```python
from build123d import *

# Parameters (mm, degrees)
SKETCH_1_W          = 25
SKETCH_1_H          = 16
EXTRUDE_1_DEPTH     = 2
SKETCH_2_R          = 0.5
CUT_EXTRUDE_1_DEPTH = 3
SKETCH_3_W          = 1.998432602
SKETCH_3_H          = 1
EXTRUDE_2_DEPTH     = 0.5
SKETCH_4_W          = 4
SKETCH_4_H          = 2
EXTRUDE_3_DEPTH     = 2
SKETCH_5_W          = 1.76862678
SKETCH_5_H          = 1.058923041
EXTRUDE_4_DEPTH     = 1


with BuildPart() as part:
    # 草图1 → 凸台-拉伸1 (new body)
    with BuildSketch(Plane.XY):
        with Locations((12.5, 8)):
            Rectangle(SKETCH_1_W, SKETCH_1_H)
    extrude(amount=EXTRUDE_1_DEPTH)

    # 草图2 → 切除-拉伸1 (cut, through all)
    with BuildSketch(Plane(origin=(0, 0, 0), x_dir=(-1, 0, 0), z_dir=(0, 0, -1))):
        with Locations((-1, 14.4)):
            Circle(SKETCH_2_R)
        with Locations((-1, 11.86)):
            Circle(SKETCH_2_R)
        with Locations((-1, 9.32)):
            Circle(SKETCH_2_R)
        with Locations((-1, 6.78)):
            Circle(SKETCH_2_R)
        with Locations((-1, 4.24)):
            Circle(SKETCH_2_R)
        with Locations((-1, 1.7)):
            Circle(SKETCH_2_R)
    extrude(amount=-CUT_EXTRUDE_1_DEPTH, mode=Mode.SUBTRACT)

    # 草图3 → 凸台-拉伸2 (add)
    with BuildSketch(Plane(origin=(0, 0, 0), x_dir=(-1, 0, 0), z_dir=(0, 0, -1))):
        with Locations((-22.800563102, 10)):
            Rectangle(SKETCH_3_W, SKETCH_3_H)
        with Locations((-22.800563102, 8)):
            Rectangle(SKETCH_3_W, SKETCH_3_H)
        with Locations((-22.800563102, 6)):
            Rectangle(SKETCH_3_W, SKETCH_3_H)
        with Locations((-22.800563102, 4)):
            Rectangle(SKETCH_3_W, SKETCH_3_H)
    extrude(amount=EXTRUDE_2_DEPTH)

    # 草图4 → 凸台-拉伸3 (add)
    with BuildSketch(Plane(origin=(0, 0, 0), x_dir=(-1, 0, 0), z_dir=(0, 0, -1))):
        with Locations((-20, 1)):
            Rectangle(SKETCH_4_W, SKETCH_4_H)
    extrude(amount=EXTRUDE_3_DEPTH)

    # 草图5 → 凸台-拉伸4 (add)
    with BuildSketch(Plane.XZ):
        with Locations((19.9984492, -0.838988802)):
            Rectangle(SKETCH_5_W, SKETCH_5_H)
    extrude(amount=EXTRUDE_4_DEPTH)


solid = part.part
```
Design review of the part built by this model. Coordinates are the model's own, in mm. A direction names the side the tool comes from. Coordinates: 2 decimals unless noted, no trailing zeros. Order: outer loops, then holes, each group sorted by start corner. A loop starts at its lowest first (then second) coordinate and runs counter-clockwise, first axis right, second up. Notation, with made-up numbers: (-19.5, 42) - (-1.5, 42) arc R14 cw to (-1.5, 61) - close; hole circle Ø5 at (15.25, 63). An arc over 180 degrees is marked (long way). Answer in a Markdown table with one row per item.
(1) Consider section B-B on z = 0.65. State the section outline as (x, y) points, plus the area to 3 significant figures.
Checked values:
| item | result |
|---|---|
| outline | (0, 0) - (25, 0) - (25, 16) - (0, 16) - close; hole circle Ø1 at (1, 1.7); hole circle Ø1 at (1, 4.24); hole circle Ø1 at (1, 6.78); hole circle Ø1 at (1, 9.32); hole circle Ø1 at (1, 11.86); hole circle Ø1 at (1, 14.4) |
| area | 395 mm^2 |
(2) For faces 1 (the flat face through (20, -0.5, -0.31)), 2 (the flat face through (20.883, -0.5, -0.8)), 3 (the flat face through (18, 1, -1)), list the 3-axis set-ups (+Z, -Z, +X, -X, +Y, -Y) from which the entire face can be reached by the end or side of a thin tool; tool diameter is ignored.
Checked values:
| item | result |
|---|---|
| face 1 | +Z, +X, -X, -Y |
| face 2 | +Z, -Z, +X, -Y |
| face 3 | -Z, -X, +Y, -Y |
(3) Wall thickness on line 1 along Y through (x, z) = (9.5, 0.6); line 2 along Z through (x, y) = (22, 4.75); line 3 along X through (y, z) = (9, 0.2): over which ranges is each line inside the solid? List them lowest first. Write a range as from..to.
Checked values:
| item | result |
|---|---|
| line 1 | 0..16 |
| line 2 | 0..2 |
| line 3 | 0..0.62, 1.38..25 |
(4) Consider section A-A on y = 1.7. State the section outline as (x, z) points, plus the area to 3 significant figures.
Checked values:
| item | result |
|---|---|
| outline | (0, 0) - (0.5, 0) - (0.5, 2) - (0, 2) - close; (1.5, 0) - (18, 0) - (18, -2) - (22, -2) - (22, 0) - (25, 0) - (25, 2) - (1.5, 2) - close |
| area | 56.0 mm^2 |
(5) Clearance check with flat-ended pins moving along their axes: pin 1 (0.5 mm diameter, centred on x = 22.5, y = 6, fed in from -Z); pin 2 (2 mm diameter, centred on x = 5, z = -0.5, fed in from -Y); pin 3 (0.8 mm diameter, centred on x = 20, y = -0.5, fed in from -Z). State where each tip first meets the part, or that it passes through.
Checked values:
| item | result |
|---|---|
| pin 1 | z = -0.5 |
| pin 2 | y = 0 |
| pin 3 | z = -1.37 |
(6) The part is to be moulded in two halves that separate along Y. For faces 4 (the cylindrical face through (1.108, 11.372, 0.986)), 5 (the flat face through (12, 16, 1)), 6 (the cylindrical face through (1.065, 7.276, 0.986)), 7 (the flat face through (0, 8, 1)), say which applies: released by +Y, released by -Y, zero draft, split by the parting line, or undercut.
Checked values:
| item | result |
|---|---|
| face 4 | undercut |
| face 5 | released by +Y |
| face 6 | undercut |
| face 7 | zero draft |
(7) Consider section D-D on y = 11.86. State the section outline as (x, z) points, plus the area to 3 significant figures.
Checked values:
| item | result |
|---|---|
| outline | (0, 0) - (0.5, 0) - (0.5, 2) - (0, 2) - close; (1.5, 0) - (25, 0) - (25, 2) - (1.5, 2) - close |
| area | 48.0 mm^2 |
(8) Consider section C-C on x = 1. State the section outline as (y, z) points, plus the area to 3 significant figures.
Checked values:
| item | result |
|---|---|
| outline | (0, 0) - (1.2, 0) - (1.2, 2) - (0, 2) - close; (2.2, 0) - (3.74, 0) - (3.74, 2) - (2.2, 2) - close; (4.74, 0) - (6.28, 0) - (6.28, 2) - (4.74, 2) - close; (7.28, 0) - (8.82, 0) - (8.82, 2) - (7.28, 2) - close; (9.82, 0) - (11.36, 0) - (11.36, 2) - (9.82, 2) - close; (12.36, 0) - (13.9, 0) - (13.9, 2) - (12.36, 2) - close; (14.9, 0) - (16, 0) - (16, 2) - (14.9, 2) - close |
| area | 20.0 mm^2 |
